Verification items for the finished model (mm, model axes). Coordinates: 2 decimals unless noted, no trailing zeros. Order: outer loops, then holes, each group sorted by start corner. A loop starts at its lowest first (then second) coordinate and runs counter-clockwise, first axis right, second up. Notation, with made-up numbers: (-35.5, 65) -> (23.5, 65) arc R21 ccw to (23.5, 83) -> close; hole circle Ø1 at (-31, 76). An arc over 180 degrees is marked (long way). Answer as CSV lines item,"result".
```python
from build123d import *

# Parameters (mm, degrees)
EXTRUDE_1_DEPTH     = 1.8
SKETCH_5_R          = 2.1
CUT_EXTRUDE_1_DEPTH = 8.195369054
HOLE_WIZARD_M5_1_D  = 4.2


with BuildPart() as part:
    # 草图1 → 凸台-拉伸1 (new body)
    with BuildSketch(Plane(origin=(0, 0, 0), x_dir=(1, 0, 0), z_dir=(0, 1, 0))):
        Polygon((4.618802154, 0), (2.309401077, 4), (-2.309401077, 4), (-4.618802154, 0), (-2.309401077, -4), (2.309401077, -4), align=None)
    extrude_1 = extrude(amount=EXTRUDE_1_DEPTH)

    # 草图4 for 放样1 → 放样1 section 0
    with BuildSketch(Plane(origin=(0, -0.1, 0), x_dir=(-1, 0, 0), z_dir=(0, -1, 0))):
        with BuildLine():
            # circular arc as an exact rational Bezier (weights 1, cos(half-angle), 1)
            Bezier((-4, 0), (-4, -2.309401077), (-2, -3.464101615), weights=[1, 0.866025404, 1])
            Bezier((-2, -3.464101615), (0, -4.618802154), (2, -3.464101615), weights=[1, 0.866025404, 1])
            Bezier((2, -3.464101615), (4, -2.309401077), (4, 0), weights=[1, 0.866025404, 1])
            Bezier((4, 0), (4, 2.309401077), (2, 3.464101615), weights=[1, 0.866025404, 1])
            Bezier((2, 3.464101615), (0, 4.618802154), (-2, 3.464101615), weights=[1, 0.866025404, 1])
            Bezier((-2, 3.464101615), (-4, 2.309401077), (-4, 0), weights=[1, 0.866025404, 1])
        make_face()
    # 草图3 → 放样1 section 1
    with BuildSketch(Plane.XZ):
        with BuildLine():
            Line((4.618802154, 0), (2.309401077, 4))
            Line((2.309401077, 4), (-2.309401077, 4))
            Line((-2.309401077, 4), (-4.618802154, 0))
            Line((-4.618802154, 0), (-2.309401077, -4))
            Line((-2.309401077, -4), (2.309401077, -4))
            Line((2.309401077, -4), (4.618802154, 0))
        make_face()
    loft_1 = loft()

    # 镜向1: 凸台-拉伸1, 放样1 across plane
    add(extrude_1.mirror(Plane.ZX.offset(1.8)))
    add(loft_1.mirror(Plane.ZX.offset(1.8)))

    # 草图5 → 切除-拉伸1 (cut, through all)
    with BuildSketch(Plane(origin=(0, -0.1, 0), x_dir=(1, 0, 0), z_dir=(0, 1, 0))):
        with Locations(Location((0, 0, 0), (0, 0, 270))):
            Circle(SKETCH_5_R)
    extrude(amount=CUT_EXTRUDE_1_DEPTH, mode=Mode.SUBTRACT)

    # M5 螺纹孔1 (through all)
    with Locations(Plane.ZX.offset(3.7)):
        with Locations((0, 0)):
            Hole(HOLE_WIZARD_M5_1_D / 2)


solid = part.part
```
Item 1: Depth check by flat-ended pin: pin 1 Ø1.5 at (y, z) = (1.5, -1) entering from -X. Enter the tip coordinate at first touch or a pass-through.
Answer list:
pin 1,"x = -4.47"
Item 2: Release check for a two-part mould opening along X. For faces 1 (the flat face through (-3.48, 1.83, 1.97)), 2 (the cylindrical face through (0.631, 1.773, 2.003)), 3 (the flat face through (0.7, -0.1, -2.4)) record: +X half, -X half, draft (parallel to the pull), parting line (faces both ways), or undercut.
Answer list:
face 1,"-X half"
face 2,"undercut"
face 3,"draft"
Item 3: Section check A-A, the plane y = 3.25. Record the boundary of the cut face in (x, z), plus the area to 3 significant figures.
Answer list:
outline,"(-4.62, 0) -> (-2.31, -4) -> (2.31, -4) -> (4.62, 0) -> (2.31, 4) -> (-2.31, 4) -> close; hole circle Ø4.2 at (0, 0)"
area,"41.6 mm2"
Item 4: Thickness scan on line 1 (Z direction, x = 0, y = 2.3); line 2 (Z direction, x = 1, y = 3.3); line 3 (X direction, y = 0.8, z = 0.25). Record the ranges inside material, lowest first.
Answer list:
line 1,"-4 to -2.1, 2.1 to 4"
line 2,"-4 to -1.85, 1.85 to 4"
line 3,"-4.47 to -2.09, 2.09 to 4.47"
